```python
from build123d import *

# Parameters (mm, degrees)
F0_W     = 62
F0_H     = 45
F1_DEPTH = 42
F3_DEPTH = 40
F5_DEPTH = 62.001
F6_R     = 2


with BuildPart() as f1:
    # F0 (on Top) → F1 (new body)
    with BuildSketch(Plane.XY):
        Rectangle(F0_W, F0_H)
    extrude(amount=F1_DEPTH)

    # F2 (on face) → F3 (cut)
    with BuildSketch(Plane.XY.offset(42)):
        Polygon((-19, -17.5), (-19, -22.5), (19, -22.5), (19, -17.5), (26, -17.5), (26, -6), (31, -6), (31, 3), (26, 3), (26, 17.5), (-26, 17.5), (-26, 3), (-31, 3), (-31, -6), (-26, -6), (-26, -17.5), align=None)
    extrude(amount=-F3_DEPTH, mode=Mode.SUBTRACT)

    # F4 (on face) → F5 (cut, through all)
    with BuildSketch(Plane.YZ.offset(31)):
        Polygon((17.5, 42), (-22.5, 42), (-22.5, 32), align=None)
    extrude(amount=-F5_DEPTH, mode=Mode.SUBTRACT)

    # F6
    f6_edges = [f1.edges().sort_by_distance(p)[0] for p in [
        (22.5, -17.5, 33.25),
        (26, -11.75, 34.6875),
        (31, -14.25, 34.0625),
        (25, -22.5, 32),
        (26, 10.25, 40.1875),
        (-26, 10.25, 40.1875),
        (-31, -14.25, 34.0625),
        (-31, 10.25, 40.1875),
        (-26, -11.75, 34.6875),
        (-22.5, -17.5, 33.25),
        (-25, -22.5, 32),
        (31, 10.25, 40.1875),
        (31, 20, 42),
        (0, 22.5, 42),
        (-31, 20, 42),
    ]]
    fillet(f6_edges, radius=F6_R)


solid = f1.part
```
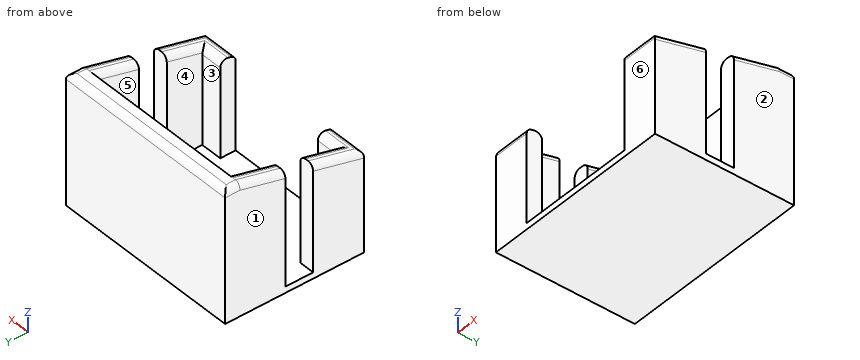
Verification items for the finished model (mm, model axes). Face numbers are marked on the shaded views. A direction names the side the tool comes from. Coordinates: 2 decimals unless noted, no trailing zeros. Loops run counter-clockwise (first coordinate to the right, second up) from the corner with the lowest first, then second, coordinate; pieces in that order, holes last. Notation, with made-up numbers: (-17, 19) - (-2, 19) arc R10 cw to (-2, 26) - close; hole circle Ø3 at (43.25, 17.25). An arc over 180 degrees is marked (long way). Return JSON: item names as keys, results as strings.
1. Section check A-A, the plane z = 8. Record the boundary of the cut face in (x, y).
Established:
{"outline": "(-31, -22.5) - (-19, -22.5) - (-19, -17.5) - (-26, -17.5) - (-26, -6) - (-31, -6) - close; (-31, 3) - (-26, 3) - (-26, 17.5) - (26, 17.5) - (26, 3) - (31, 3) - (31, 22.5) - (-31, 22.5) - close; (19, -22.5) - (31, -22.5) - (31, -6) - (26, -6) - (26, -17.5) - (19, -17.5) - close"}
2. Go/stop test with a flat-tipped pin: pin 1 (4 mm diameter, centred on x = 7, y = 15, fed in from +Z). Record where the tip stops, or that it passes through.
Established:
{"pin 1": "stops at z = 2"}
3. Mould release check, pull along X, two halves, no side actions. Record for the marked faces 1, 2, 3 and 4: +X half, -X half, draft (parallel to the pull), parting line (faces both ways), or undercut.
Established:
{"face 1": "-X half", "face 2": "+X half", "face 3": "undercut", "face 4": "undercut"}
4. Section check B-B, the plane x = 0.5. Record the boundary of the cut face in (y, z), then the cut area to 3 significant figures.
Established:
{"outline": "(-22.5, 0) - (22.5, 0) - (22.5, 40) arc R2 ccw to (20.5, 42) - (17.5, 42) - (17.5, 2) - (-22.5, 2) - close", "area": "289 mm2"}
5. Section check C-C, the plane y = 1. Record the boundary of the cut face in (x, z), then the cut area to 3 significant figures.
Established:
{"outline": "(-31, 0) - (31, 0) - (31, 2) - (-31, 2) - close", "area": "124 mm2"}
6. Thickness scan on L1, parallel to X at y = 17, z = 12; L2, parallel to Y at x = -10.5, z = 33.5; L3, parallel to Z at x = -2.5, y = 12. Record the ranges inside material, lowest first.
Established:
{"L1": "x = -31 to -26, 26 to 31", "L2": "y = 17.5 to 22.5", "L3": "z = 0 to 2"}
7. Tool access check on the marked faces 5 and 6. Record the directions out of +Z, -Z, +X, -X, +Y, -Y that give a thin tool (end or side, any length) a straight path to the whole face; none if there is none.
Established:
{"face 5": "+Z", "face 6": "+Z, -Z, +X, -X, -Y"}
